from build123d import *

# Parameters (mm, degrees)
BASPROSKE_W                = 9
BASPROSKE_H                = 45
TOOTHCUT_DEPTH             = 65.272855857
TEETHCUTS_COUNT            = 43
TEETHCUTS_ANGLE            = 351.627906977
BORSKE_R                   = 3
BORE_DEPTH                 = 50.0000508
WYTNIJ_WYCI_GNI_CIE1_DEPTH = 65.265003825


with BuildPart() as part:
    # BasProSke → Base-Revolve (revolve)
    with BuildSketch(Plane(origin=(0, 0, 0), x_dir=(1, 0, 0), z_dir=(0, 1, 0)), mode=Mode.PRIVATE) as base_revolve_sk:
        with Locations((4.5, 22.5)):
            Rectangle(BASPROSKE_W, BASPROSKE_H)
    revolve(base_revolve_sk.sketch.rotate(Axis((-10, 0, 0), (1, 0, 0)), 180), axis=Axis((-10, 0, 0), (1, 0, 0)))

    # TooCutSke → ToothCut (cut, through all)
    with BuildSketch(Plane(origin=(0, 0, 0), x_dir=(0, 0, -1), z_dir=(1, 0, 0))):
        with BuildLine():
            ThreePointArc((0.875138877, 40.489543501), (0, 40.499), (-0.875138877, 40.489543501))
            ThreePointArc((-0.875138877, 40.489543501), (-1.611840844, 42.780747503), (-2.66114443, 44.94669015))
            ThreePointArc((-2.66114443, 44.94669015), (0, 45.0254), (2.66114443, 44.94669015))
            ThreePointArc((2.66114443, 44.94669015), (1.611840844, 42.780747503), (0.875138877, 40.489543501))
        make_face()
    toothcut = extrude(amount=TOOTHCUT_DEPTH, mode=Mode.SUBTRACT)

    # TeethCuts: ToothCut ×43 about axis
    teethcuts_axis = Axis((-10, 0, 0), (1, 0, 0))
    for i in range(1, TEETHCUTS_COUNT):
        add(toothcut.rotate(teethcuts_axis, i * TEETHCUTS_ANGLE / (TEETHCUTS_COUNT - 1)), mode=Mode.SUBTRACT)

    # BorSke → Bore (cut, symmetric)
    with BuildSketch(Plane(origin=(0, 0, 0), x_dir=(0, 0, -1), z_dir=(1, 0, 0))):
        with Locations(Location((0, 0, 0), (0, 0, 180))):
            Circle(BORSKE_R)
    extrude(amount=BORE_DEPTH, both=True, mode=Mode.SUBTRACT)

    # Szkic2 → Wytnij-wyciągnięcie1 (cut, through all)
    with BuildSketch(Plane(origin=(0, 0, 0), x_dir=(0, 0, -1), z_dir=(1, 0, 0))):
        with BuildLine():
            Line((-31.467717921, -38.8559227), (-22.027402545, -27.19914589))
            ThreePointArc((-22.027402545, -27.19914589), (30.975282492, -16.295148804), (9.936124572, 33.559997445))
            Line((9.936124572, 33.559997445), (14.194463674, 47.942853492))
            ThreePointArc((14.194463674, 47.942853492), (-44.25040356, 23.278784006), (-31.467717921, -38.8559227))
        make_face()
    extrude(amount=WYTNIJ_WYCI_GNI_CIE1_DEPTH, mode=Mode.SUBTRACT)


solid = part.part
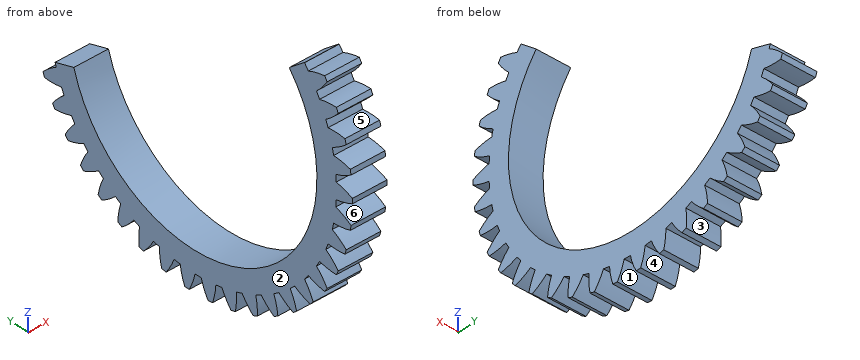
Geometry check sheet. Reference: the model listing, model coordinates, mm. Face numbers are marked on the shaded views. A direction names the side the tool comes from. Round coordinates to 2 decimals unless told otherwise and drop trailing zeros.
Item 1: Access from +Z, -Z, +X, -X, +Y, -Y to the whole of each face (thin tool, end or side, straight path). Record for the marked faces 4, 5 and 6.
Item 2: Gauge pin test, flat ends, axial feed: pin 1 (2 mm diameter, centred on x = 4.5, z = 0, fed in from +Y); pin 2 (1 mm diameter, centred on x = 1.5, y = -32.5, fed in from -Z); pin 3 (1 mm diameter, centred on x = 4.5, z = -7, fed in from -Y). Record the tip position at first contact, or that the pin passes through.
Item 3: Thickness scan on line 1 (Y direction, x = 3.25, z = -13.5); line 2 (Y direction, x = 7.75, z = -12); line 3 (Y direction, x = 3, z = 0). Record the ranges inside material, lowest first.
Item 4: Mould release check, pull along Z, two halves, no side actions. Record for the marked faces 1, 2 and 3: pulls with the +Z half, pulls with the -Z half, needs draft (parallel to the pull), parting line crosses it, or undercut.
Answer sheet:
1. face 4: -Z, +X, -X
1. face 5: +X, -X
1. face 6: +X, -X, -Y
2. pin 1: stops at y = -34.99
2. pin 2: stops at z = -30.48
2. pin 3: stops at y = -44.53
3. line 1: y = -42.93 to -32.29, 32.29 to 40.02
3. line 2: y = -42.87 to -32.88, 32.88 to 38.68
3. line 3: y = -45 to -35
4. face 1: pulls with the -Z half
4. face 2: needs draft
4. face 3: undercut
